```python
from build123d import *

# Parameters (mm, degrees)
F0_W      = 96
F0_H      = 78
F1_DEPTH  = 18
F2_W      = 72
F2_H      = 38
F4_DEPTH  = 58
F6_DEPTH  = 38
F8_DEPTH  = 72.001
F9_W      = 8
F9_H      = 12
F10_DEPTH = 60.001
F12_DEPTH = 3
F14_DEPTH = 21
F15_W     = 20
F15_H     = 5
F16_DEPTH = 96.001
F17_W     = 3
F17_H     = 14
F18_DEPTH = 72
F19_R     = 2.99999


# Not quite as in the source:
# - a fillet or chamfer is up to 0.001 mm smaller than in the source, because OpenCascade refuses the exact size


with BuildPart() as f1:
    # F0 (on Top) → F1 (new body)
    with BuildSketch(Plane.XY):
        with Locations((48, 39)):
            Rectangle(F0_W, F0_H)
    extrude(amount=F1_DEPTH)

    # F2 (on face) → F4 (join, through all)
    with BuildSketch(Plane.XY.offset(18)):
        with Locations((48, 59)):
            Rectangle(F2_W, F2_H)
    extrude(amount=F4_DEPTH)

    # F5 (on face) → F6 (cut, through all)
    with BuildSketch(Plane.XZ.offset(-40)):
        Polygon((84, 76), (60, 76), (84, 52), align=None)
    extrude(amount=-F6_DEPTH, mode=Mode.SUBTRACT)

    # F7 (on face) → F8 (cut, through all)
    with BuildSketch(Plane(origin=(12, 0, 0), x_dir=(0, -1, 0), z_dir=(-1, 0, 0))):
        Polygon((-78, 76), (-78, 40), (-64, 76), align=None)
    extrude(amount=-F8_DEPTH, mode=Mode.SUBTRACT)

    # F9 (on face) → F10 (cut, through all)
    with BuildSketch(Plane(origin=(12, 0, 0), x_dir=(0, -1, 0), z_dir=(-1, 0, 0))):
        with Locations((-52, 70)):
            Rectangle(F9_W, F9_H)
    extrude(amount=-F10_DEPTH, mode=Mode.SUBTRACT)

    # F11 (on face) → F12 (join)
    with BuildSketch(Plane.XY.offset(18)):
        with BuildLine():
            Line((71, 33), (25, 33))
            ThreePointArc((25, 33), (12, 20), (25, 7))
            Line((25, 7), (71, 7))
            ThreePointArc((71, 7), (84, 20), (71, 33))
        make_face()
    extrude(amount=F12_DEPTH)

    # F13 (on face) → F14 (cut, through all)
    with BuildSketch(Plane.XY.offset(21)):
        with BuildLine():
            Line((71, 26), (25, 26))
            ThreePointArc((25, 26), (19, 20), (25, 14))
            Line((25, 14), (71, 14))
            ThreePointArc((71, 14), (77, 20), (71, 26))
        make_face()
    extrude(amount=-F14_DEPTH, mode=Mode.SUBTRACT)

    # F15 (on face) → F16 (cut, through all)
    with BuildSketch(Plane.YZ.offset(96)):
        with Locations((20, 2.5)):
            Rectangle(F15_W, F15_H)
    extrude(amount=-F16_DEPTH, mode=Mode.SUBTRACT)

    # F17 (on face) → F18 (cut, through all)
    with BuildSketch(Plane.YZ.offset(84)):
        with Locations((41.5, 25)):
            Rectangle(F17_W, F17_H)
    extrude(amount=-F18_DEPTH, mode=Mode.SUBTRACT)

    # F19 (radius 3 in the source; OpenCascade refuses exactly that, so slightly less here)
    f19_edges = [f1.edges().sort_by_distance(p)[0] for p in [
        (48, 43, 18),
        (48, 43, 32),
        (96, 39, 18),
        (48, 0, 18),
        (96, 0, 9),
        (96, 78, 9),
        (90, 78, 18),
        (0, 39, 18),
        (0, 0, 9),
        (0, 78, 9),
        (6, 78, 18),
    ]]
    fillet(f19_edges, radius=F19_R)


solid = f1.part
```
Input: part model. Units: mm. Frame: model coordinates. A direction names the side the tool comes from. Give positions to 0.01 mm unless a question says otherwise; leave off trailing zeros. Loops run counter-clockwise (first coordinate to the right, second up) from the corner with the lowest first, then second, coordinate; pieces in that order, holes last. Notation, with made-up numbers: (6, -39) -> (34, -39) arc R14 cw to (34, -19) -> close; hole circle Ø4 at (-25, 35.25). An arc over 180 degrees is marked (long way). Use a Markdown table: item, result.
Q1. Section query C-C, the plane y = 59.5. Return the cut outline in (x, z).
Entries:
| item | result |
|---|---|
| outline | (0, 0) -> (96, 0) -> (96, 15) arc R3 ccw to (93, 18) -> (84, 18) -> (84, 52) -> (60, 76) -> (12, 76) -> (12, 18) -> (3, 18) arc R3 ccw to (0, 15) -> close |
Q2. Section query A-A, the plane y = 20. Return the cut outline in (x, z), plus the area to 3 significant figures.
Entries:
| item | result |
|---|---|
| outline | (0, 5) -> (19, 5) -> (19, 21) -> (12, 21) -> (12, 18) -> (3, 18) arc R3 ccw to (0, 15) -> close; (77, 5) -> (96, 5) -> (96, 15) arc R3 ccw to (93, 18) -> (84, 18) -> (84, 21) -> (77, 21) -> close |
| area | 532 mm² |
Q3. Section query B-B, the plane x = 6.5. Return the cut outline in (y, z), plus the area to 3 significant figures.
Entries:
| item | result |
|---|---|
| outline | (0, 0) -> (10, 0) -> (10, 5) -> (30, 5) -> (30, 0) -> (78, 0) -> (78, 15) arc R3 ccw to (75, 18) -> (3, 18) arc R3 ccw to (0, 15) -> close |
| area | 1,300 mm² |
Q4. First-contact query: P1, Ø1, axis at x = 53, z = 27, coming from the -Y side; P2, Ø8, axis at x = 36, z = 30, coming from the -Y side; P3, Ø1, axis at x = 12.5, y = 35, coming from the +Z side. Flat tips, straight axial feed; report the tip coordinate or a pass-through.
Entries:
| item | result |
|---|---|
| P1 | stops at y = 43 |
| P2 | stops at y = 40 |
| P3 | stops at z = 18 |
Q5. Ray query, probe 1 along Y at (x, z) = (44, 6.5); probe 2 along X at (y, z) = (42.5, 44); probe 3 along Z at (x, y) = (5.5, 17). Return the intervals inside material, ascending. Write a range as from..to.
Entries:
| item | result |
|---|---|
| probe 1 | y = 0..14, 26..78 |
| probe 2 | x = 12..84 |
| probe 3 | z = 5..18 |
Q6. Access query for faces 1 (the cylindrical face through (12, 20, 19)), 2 (the cylindrical face through (47.5, 42.1, 18.86)), 3 (the flat face through (42, 56, 70)), 4 (the cylindrical face through (77, 20, 13)). Directions: +Z, -Z, +X, -X, +Y, -Y. A direction counts if a zero-diameter tool reaches every point of the face in a straight line with its end or side. Return the directions, or none.
Entries:
| item | result |
|---|---|
| face 1 | +Z, -X |
| face 2 | +X, -X |
| face 3 | +Z, +X, -X |
| face 4 | +Z, -Z |
Q7. Pull-direction query (X, two-part tool) for faces 5 (the flat face through (74, 56, 62)), 6 (the flat face through (48, 7, 19)), 7 (the flat face through (48, 14, 13)), 8 (the flat face through (0, 38, 7)); classes: pulls with the +X half, pulls with the -X half, needs draft (parallel to the pull), parting line crosses it, or undercut.
Entries:
| item | result |
|---|---|
| face 5 | pulls with the +X half |
| face 6 | needs draft |
| face 7 | undercut |
| face 8 | pulls with the -X half |
